Check sheet for the drawn part. Datum: minimum x, y, z corner. Units: mm. Coordinates: 2 decimals unless noted, no trailing zeros. Write each loop counter-clockwise with the first axis right and the second up, starting at its lowest first coordinate (ties: lowest second). Pieces come first, ordered by that corner, then holes. Notation, with made-up numbers: (77.25, -17.75) -> (120.25, -17.75) arc R18 cw to (120.25, 10.25) -> close; hole circle Ø8 at (2.25, -31.5). An arc over 180 degrees is marked (long way). Answer in a Markdown table with one row per item. Add a question column.
1. Cross-section at B-B on x = 102.5. Record the cut outline in (y, z).
2. Mould release check, pull along X, two halves, no side actions. Record for the marked faces 1 and 2: pulls with the +X half, pulls with the -X half, needs draft (parallel to the pull), parting line crosses it, or undercut.
3. Scan lines: L1, parallel to Y at x = 20, z = 2.8 (1 decimal); L2, parallel to Z at x = 54, y = 46; L3, parallel to Y at x = 103.5, z = 1.9. Record each from-to range of solid material in increasing order. Write a range as from..to.
4. Depth check by flat-ended pin: P1, Ø0.5, axis at x = 47.5, z = 2.5, coming from the -Y side (1 decimal); P2, Ø1, axis at y = 14.5, z = 2.5, coming from the -X side; P3, Ø0.5, axis at y = 35, z = 2.5, coming from the -X side. Enter the tip coordinate at first touch or a pass-through.
5. Cross-section at A-A on y = 44.5. Record the cut outline in (x, z) (1 decimal).
6. Cross-section at D-D on x = 75. Record the cut outline in (y, z).
7. Cross-section at C-C on z = 0.8. Record the cut outline in (x, y) (1 decimal).
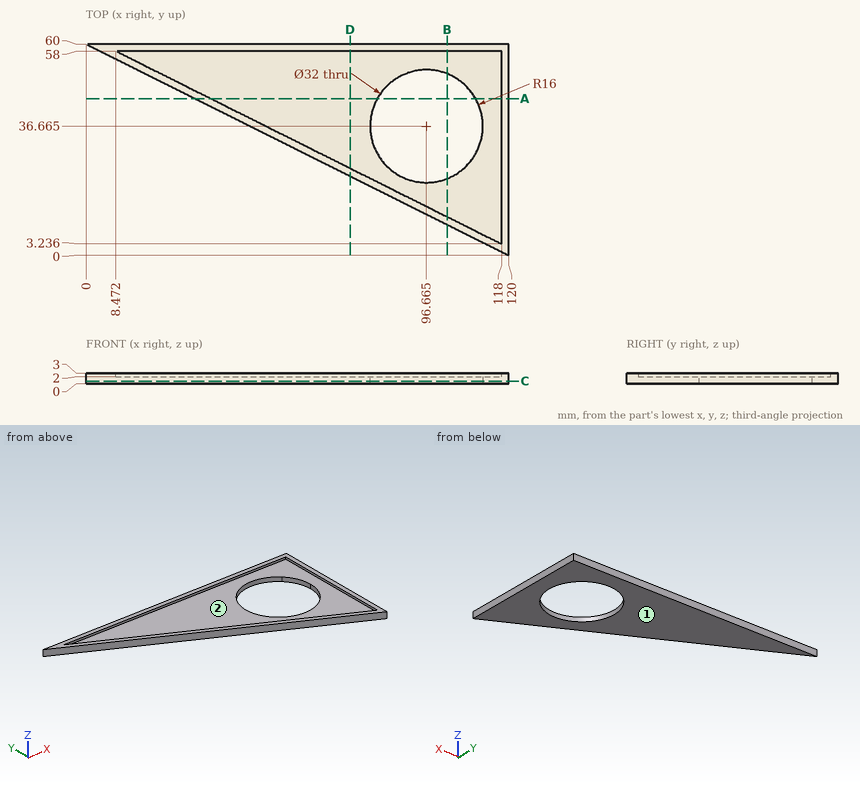
Results found:
| question | item | result |
|---|---|---|
| 1 | outline | (8.75, 0) -> (21.77, 0) -> (21.77, 2) -> (10.99, 2) -> (10.99, 3) -> (8.75, 3) -> close; (51.56, 0) -> (60, 0) -> (60, 3) -> (58, 3) -> (58, 2) -> (51.56, 2) -> close |
| 2 | face 1 | needs draft |
| 2 | face 2 | undercut |
| 3 | L1 | y = 50..52.2, 58..60 |
| 3 | L2 | z = 0..2 |
| 3 | L3 | y = 8.25..22.2, 51.13..60 |
| 4 | P1 | stops at y = 36.1 |
| 4 | P2 | stops at x = 90 |
| 4 | P3 | stops at x = 49.5 |
| 5 | outline | (31, 0) -> (82.7, 0) -> (82.7, 2) -> (35.5, 2) -> (35.5, 3) -> (31, 3) -> close; (110.6, 0) -> (120, 0) -> (120, 3) -> (118, 3) -> (118, 2) -> (110.6, 2) -> close |
| 6 | outline | (22.5, 0) -> (60, 0) -> (60, 3) -> (58, 3) -> (58, 2) -> (24.74, 2) -> (24.74, 3) -> (22.5, 3) -> close |
| 7 | outline | (0, 60) -> (120, 0) -> (120, 60) -> close; hole circle Ø32 at (96.7, 36.7) |
